from build123d import *

# Parameters (mm, degrees)
F0_W                 = 65
F0_H                 = 32
F1_DEPTH             = 14.25
F4_D                 = 9
F4_DEPTH             = 40
F4_CBORE_D           = 15
F4_CBORE_DEPTH       = 12
F4_TIP               = 2.7038727856
F4_ON_F3_D           = 9
F4_ON_F3_DEPTH       = 40
F4_ON_F3_CBORE_D     = 15
F4_ON_F3_CBORE_DEPTH = 12
F4_ON_F3_TIP         = 2.7038727856
F5_R                 = 1.5


with BuildPart() as f1:
    # F0 (on Front) → F1 (new body, symmetric)
    with BuildSketch(Plane.XZ):
        Rectangle(F0_W, F0_H)
    extrude(amount=F1_DEPTH, both=True)

    # F4
    with Locations(Plane.XY.offset(16)):
        with Locations((-18, 0), (18, 0)):
            CounterBoreHole(F4_D / 2, F4_CBORE_D / 2, F4_CBORE_DEPTH, depth=F4_DEPTH)
            with Locations((0, 0, -(F4_DEPTH + F4_TIP / 2))):  # 118° drill point
                Cone(0, F4_D / 2, F4_TIP, mode=Mode.SUBTRACT)

    # F4 on F3
    with Locations(Plane(origin=(0, 0, -16), x_dir=(1, 0, 0), z_dir=(0, 0, -1))):
        with Locations((0, 0)):
            CounterBoreHole(F4_ON_F3_D / 2, F4_ON_F3_CBORE_D / 2, F4_ON_F3_CBORE_DEPTH, depth=F4_ON_F3_DEPTH)
            with Locations((0, 0, -(F4_ON_F3_DEPTH + F4_ON_F3_TIP / 2))):  # 118° drill point
                Cone(0, F4_ON_F3_D / 2, F4_ON_F3_TIP, mode=Mode.SUBTRACT)

    # F5
    f5_edges = [f1.edges().sort_by_distance(p)[0] for p in [
        (-32.5, -14.25, 0),
        (32.5, -14.25, 0),
        (32.5, 14.25, 0),
        (-32.5, 14.25, 0),
    ]]
    fillet(f5_edges, radius=F5_R)


solid = f1.part
Read the model definition and answer for the solid it produces. Units are mm, in the model's axes. A direction names the side the tool comes from. Give positions to 0.01 mm unless a question says otherwise; leave off trailing zeros. Loops run counter-clockwise (first coordinate to the right, second up) from the corner with the lowest first, then second, coordinate; pieces in that order, holes last. Notation, with made-up numbers: (53.5, -12.5) -> (100.5, -12.5) arc R31 ccw to (100.5, 18.5) -> close; hole circle Ø5 at (-12, 61). An arc over 180 degrees is marked (long way). Use a Markdown table: item, result.
Q1. Section A-A, the plane x = -18 is taken. Determine the outline of the cut face in (y, z).
Solved:
| item | result |
|---|---|
| outline | (-14.25, -16) -> (-4.5, -16) -> (-4.5, 4) -> (-7.5, 4) -> (-7.5, 16) -> (-14.25, 16) -> close; (4.5, -16) -> (14.25, -16) -> (14.25, 16) -> (7.5, 16) -> (7.5, 4) -> (4.5, 4) -> close |
Q2. A tool of negligible diameter and unlimited length cuts with its end or side. For faces 4 (the face through (0, 14.25, 0)), 5 (the face through (-7.493, -0.33, -10.084)), 6 (the face through (10.507, 0.33, 10.084)), from which of +Z, -Z, +X, -X, +Y, -Y can it reach the whole face along a straight path? Write none if from no direction.
Solved:
| item | result |
|---|---|
| face 4 | +Z, -Z, +X, -X, +Y |
| face 5 | -Z |
| face 6 | +Z |
Q3. Determine the mould class of faces 1 (the face through (-8, 0, -16)), 2 (the face through (-25.493, 0.33, 10.084)), 3 (the face through (32.5, 0, 0)) for opening direction X: pulls with the +X half, pulls with the -X half, needs draft (parallel to the pull), parting line crosses it, or undercut.
Solved:
| item | result |
|---|---|
| face 1 | needs draft |
| face 2 | undercut |
| face 3 | pulls with the +X half |
Q4. Find the intervals of material crossed by line 1 along X through (y, z) = (6, 15); line 2 along Y through (x, z) = (18, -10); line 3 along Z through (x, y) = (12, -1), in increasing order.
Solved:
| item | result |
|---|---|
| line 1 | x = -32.5 to -22.5, -13.5 to 13.5, 22.5 to 32.5 |
| line 2 | y = -14.25 to -4.5, 4.5 to 14.25 |
| line 3 | z = -16 to 4 |
Q5. Each of these flat-tipped pins is pushed along its axis until it touches: pin 1 (11.5 mm diameter, centred on x = 18, y = 0, fed in from +Z); pin 2 (5.5 mm diameter, centred on x = -18, y = 0, fed in from -Z); pin 3 (12 mm diameter, centred on x = 0, y = 0, fed in from -Z). Where does it stop, or does it pass through?
Solved:
| item | result |
|---|---|
| pin 1 | stops at z = 4 |
| pin 2 | passes through |
| pin 3 | stops at z = -4 |
Q6. Section B-B, the plane z = 10.5 is taken. Determine the outline of the cut face in (x, y).
Solved:
| item | result |
|---|---|
| outline | (-32.5, -12.75) arc R1.5 ccw to (-31, -14.25) -> (31, -14.25) arc R1.5 ccw to (32.5, -12.75) -> (32.5, 12.75) arc R1.5 ccw to (31, 14.25) -> (-31, 14.25) arc R1.5 ccw to (-32.5, 12.75) -> close; hole circle Ø15 at (-18, 0); hole circle Ø9 at (0, 0); hole circle Ø15 at (18, 0) |
Q7. Section C-C, the plane y = 3.5 is taken. Determine the outline of the cut face in (x, z), then the cut area to 3 significant figures.
Solved:
| item | result |
|---|---|
| outline | (-32.5, -16) -> (-20.83, -16) -> (-20.83, 4) -> (-24.63, 4) -> (-24.63, 16) -> (-32.5, 16) -> close; (-15.17, -16) -> (-6.63, -16) -> (-6.63, -4) -> (-2.83, -4) -> (-2.83, 16) -> (-11.37, 16) -> (-11.37, 4) -> (-15.17, 4) -> close; (2.83, -4) -> (6.63, -4) -> (6.63, -16) -> (15.17, -16) -> (15.17, 4) -> (11.37, 4) -> (11.37, 16) -> (2.83, 16) -> close; (20.83, -16) -> (32.5, -16) -> (32.5, 16) -> (24.63, 16) -> (24.63, 4) -> (20.83, 4) -> close |
| area | 1,260 mm^2 |
Q8. Section D-D, the plane z = -8.5 is taken. Determine the outline of the cut face in (x, y).
Solved:
| item | result |
|---|---|
| outline | (-32.5, -12.75) arc R1.5 ccw to (-31, -14.25) -> (31, -14.25) arc R1.5 ccw to (32.5, -12.75) -> (32.5, 12.75) arc R1.5 ccw to (31, 14.25) -> (-31, 14.25) arc R1.5 ccw to (-32.5, 12.75) -> close; hole circle Ø9 at (-18, 0); hole circle Ø15 at (0, 0); hole circle Ø9 at (18, 0) |
